CAD build for the part. Positions are in the model's coordinates, mm. Give positions to 0.01 mm unless a question says otherwise; leave off trailing zeros. Loops run counter-clockwise (first coordinate to the right, second up) from the corner with the lowest first, then second, coordinate; pieces in that order, holes last. Notation, with made-up numbers: M 52,77.25 L 58,77.25 A27 ccw 58,103.25 Z; hole C 19,-18 d6. An arc over 180 degrees is marked long. Answer as CSV lines item,"result".
```python
from build123d import *

# Parameters (mm, degrees)
F0_W     = 40
F0_H     = 1.175
F0_H_2   = 0.65
F1_DEPTH = 20
F2_DEPTH = 10


with BuildPart() as f1:
    # F0 (on Top) → F1 (new body)
    with BuildSketch(Plane.XY):
        with Locations((0, -0.9125)):
            Rectangle(F0_W, F0_H)
        Rectangle(F0_W, F0_H_2)
        with Locations((0, 0.9125)):
            Rectangle(F0_W, F0_H)
    extrude(amount=-F1_DEPTH)

    # F0 (on Top) → F2 (cut)
    with BuildSketch(Plane.XY):
        Rectangle(F0_W, F0_H_2)
    extrude(amount=-F2_DEPTH, mode=Mode.SUBTRACT)


solid = f1.part
```
Q1. Cut at A-A (z = -5.5). Write the cut outline in (x, y) (3 decimals), and give its area (3 significant figures).
Solution:
outline,"M -20,-1.5 L 20,-1.5 L 20,-0.325 L -20,-0.325 Z; M -20,0.325 L 20,0.325 L 20,1.5 L -20,1.5 Z"
area,"94.0 mm²"
Q2. Wall check: line 1 (Y direction, x = -1.5, z = -1.25) (3 decimals); line 2 (Z direction, x = -7, y = -0.1). Give the ranges that are in metal, low to high. Write a range as [from, to].
Solution:
line 1,"y = [-1.5, -0.325], [0.325, 1.5]"
line 2,"z = [-20, -10]"
Q3. Cut at B-B (x = -7). Write the cut outline in (y, z) (3 decimals), and give its area (3 significant figures).
Solution:
outline,"M -1.5,-20 L 1.5,-20 L 1.5,0 L 0.325,0 L 0.325,-10 L -0.325,-10 L -0.325,0 L -1.5,0 Z"
area,"53.5 mm²"
Q4. Mould opens along Y. For faces 1 (the flat face through (0, 1, 0)), 2 (the flat face through (0, 0.325, -5)), 3 (the flat face through (0, -1.5, -10)), 4 (the flat face through (0, -0.325, -5)) say: released by +Y, released by -Y, zero draft, split by the parting line, or undercut.
Solution:
face 1,"zero draft"
face 2,"undercut"
face 3,"released by -Y"
face 4,"undercut"
